Here's how the part is built. I have some questions about the finished solid (model axes, mm). Give positions to 0.01 mm unless a question says otherwise; leave off trailing zeros. Order: outer loops, then holes, each group sorted by start corner. A loop starts at its lowest first (then second) coordinate and runs counter-clockwise, first axis right, second up.
Autodesk Inventor part; units mm, degrees
ref_plane "YZ Plane" through (0, 0, 0) normal (1, 0, 0) x (0, 1, 0)
ref_plane "XZ Plane" through (0, 0, 0) normal (0, 1, 0) x (-1, 0, 0)
ref_plane "XY Plane" through (0, 0, 0) normal (0, 0, 1) x (1, 0, 0)
sketch "Sketch1" plane through (0, 0, 0) normal (0, 0, 1) x (1, 0, 0)
  circle A0 centre (0, 0) radius 2.25
  circle A1 centre (-10, 0) radius 2.25
  line L0 (-10, 0) -> (0, 0) construction
  line L1 (-15, 10) -> (-15, -10)
  line L2 (-15, -10) -> (25, -10)
  line L3 (-10, 0) -> (-15, 0) construction
  line L4 (-15, 10) -> (25, 10)
  circle A2 centre (20, 0) radius 2.25
  line L5 (20, 0) -> (0, 0) construction
  line L6 (20, 0) -> (25, 0) construction
  line L7 (25, 10) -> (25, -10)
  dimension "d0" = 4.5
  dimension "d1" = 10
  dimension "d2" = 5
  dimension "d3" = 20
  dimension "d4" = 4.5
  dimension "d5" = 20
  dimension "d6" = 5
extrude "Extrusion1" add sketch "Sketch1" along normal blind 5
properties part number "Y Bearing Tensioner"
Q1. If we section it at B-B on z = 0.4: List the corners of the cut face in (x, y) for me.
Filled sheet:
outline: (-15, -10) - (25, -10) - (25, 10) - (-15, 10) - close; hole circle Ø4.5 at (-10, 0); hole circle Ø4.5 at (0, 0); hole circle Ø4.5 at (20, 0)
Q2. Thinking about a two-plate mould opening in X: for faces 1 (the face through (-15, 0, 2)), 2 (the face through (-0.29, -2.23, 2.46)), 3 (the face through (5, 0, 0)), which applies, released by +X, released by -X, zero draft, split by the parting line, or undercut?
Filled sheet:
face 1: released by -X
face 2: undercut
face 3: zero draft
Q3. I'm going to push a flat-ended pin straight in: P1, Ø4, axis at x = 20, y = 0, coming from the -Z side. Where does the tip first touch, or does it pass through?
Filled sheet:
P1: passes through
Q4. If we section it at C-C on y = -0.75: List the corners of the cut face in (x, z) for me.
Filled sheet:
outline: (-15, 0) - (-12.12, 0) - (-12.12, 5) - (-15, 5) - close; (-7.88, 0) - (-2.12, 0) - (-2.12, 5) - (-7.88, 5) - close; (2.12, 0) - (17.88, 0) - (17.88, 5) - (2.12, 5) - close; (22.12, 0) - (25, 0) - (25, 5) - (22.12, 5) - close
Q5. I need wall thicknesses on L1, parallel to Y at x = 20, z = 3.55; L2, parallel to Y at x = -9, z = 2.3; L3, parallel to X at y = -2, z = 0.45. Which ranges of each line are inside material? Lowest first, please.
Filled sheet:
L1: y = -10 to -2.25, 2.25 to 10
L2: y = -10 to -2.02, 2.02 to 10
L3: x = -15 to -11.03, -8.97 to -1.03, 1.03 to 18.97, 21.03 to 25
Q6. If we section it at A-A on x = -10: List the corners of the cut face in (y, z) for me, plus the area to 3 significant figures.
Filled sheet:
outline: (-10, 0) - (-2.25, 0) - (-2.25, 5) - (-10, 5) - close; (2.25, 0) - (10, 0) - (10, 5) - (2.25, 5) - close
area: 77.5 mm2
Q7. If we section it at D-D on x = 0.5: List the corners of the cut face in (y, z) for me.
Filled sheet:
outline: (-10, 0) - (-2.19, 0) - (-2.19, 5) - (-10, 5) - close; (2.19, 0) - (10, 0) - (10, 5) - (2.19, 5) - close
